Autodesk Inventor part; units mm, degrees
ref_plane "YZ Plane" through (0, 0, 0) normal (1, 0, 0) x (0, 1, 0)
ref_plane "XZ Plane" through (0, 0, 0) normal (0, 1, 0) x (-1, 0, 0)
ref_plane "XY Plane" through (0, 0, 0) normal (0, 0, 1) x (1, 0, 0)
sketch "Esboço1" plane through (0, 0, 0) normal (0, 1, 0) x (-1, 0, 0)
  circle A0 centre (0, 0) radius 15
  dimension "d0" = 30
extrude "Extrusão1" add sketch "Esboço1" along normal mid plane 21.5
fillet "Arredondamento1" radius 2 1 edges at (15, 10.75, 0)
sketch "Esboço2" plane through (0, -10.75, 0) normal (0, -1, 0) x (1, 0, 0)
  circle A0 centre (0, 0) radius 5
  dimension "d4" = 10
extrude "Extrusão2" cut sketch "Esboço2" against normal blind 10
sketch "Esboço3" plane through (0, 10.75, 0) normal (0, 1, 0) x (1, 0, 0)
  line L0 (2.5, -7.5) -> (-2.5, -7.5)
  line L1 (-2.5, -7.5) -> (-2.5, 7.5)
  line L2 (-2.5, 7.5) -> (2.5, 7.5)
  line L3 (2.5, 7.5) -> (2.5, -7.5)
  line L4 (2.5, -7.5) -> (-2.5, 7.5) construction
  line L5 (-2.5, -7.5) -> (2.5, 7.5) construction
  point P0 (0, 0)
  dimension "d7" = 5
  dimension "d8" = 15
extrude "Extrusão3" add sketch "Esboço3" along normal blind 44.25
fillet "Arredondamento2" radius 7.5 1 edges at (0, 55, 7.5)
fillet "Arredondamento3" radius 7.5 1 edges at (0, 55, -7.5)
fillet "Arredondamento4" radius 2 1 edges at (2.5, 10.75, 0)
fillet "Arredondamento5" radius 2 1 edges at (-2.5, 10.75, 0)
sketch "Esboço4" plane through (2.5, 47.5, 0) normal (1, 0, 0) x (0, 0, -1)
  line L0 (-7.5, -34.75) -> (-7.5, 0)
  line L1 (7.5, -34.75) -> (7.5, 0)
  line L2 (-7.5, 0) -> (7.5, 0) construction
  circle A0 centre (0, 0) radius 4
  point P0 (0, -47.5)
  dimension "d15" = 8
extrude "Extrusão4" add sketch "Esboço4" along normal blind 5.5
fillet "Arredondamento6" radius 0.5 1 edges at (8, 47.5, 4)
properties part number "Corpo do robo"
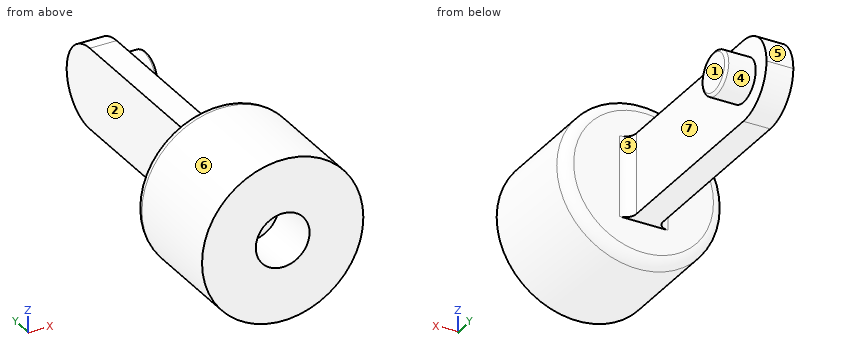
Could you check a few things on this model? Use its own coordinates, in mm. Face numbers are marked on the shaded views. A direction names the side the tool comes from. Coordinates: 2 decimals unless noted, no trailing zeros. Loops run counter-clockwise (first coordinate to the right, second up) from the corner with the lowest first, then second, coordinate; pieces in that order, holes last. Notation, with made-up numbers: (4, 70) -> (63, 70) arc R29 ccw to (63, 93) -> close; hole circle Ø11 at (-5, 31). An arc over 180 degrees is marked (long way). Answer in a Markdown table with one row per item.
(1) If I drill on probe 1 along Z at (x, y) = (0, -3); probe 2 along Y at (x, z) = (10.75, 3.5); probe 3 along Z at (x, y) = (-1, 18.5), over which ranges is the centre line in solid material (lowest first)?
Results found:
| item | result |
|---|---|
| probe 1 | z = -15 to -5, 5 to 15 |
| probe 2 | y = -10.75 to 10.75 |
| probe 3 | z = -7.5 to 7.5 |
(2) Will these pins go through, and if not, where does the flat tip stop? pin 1 Ø6 at (x, z) = (-2.5, 1.5) entering from +Y; pin 2 Ø5.5 at (y, z) = (46, 0.5) entering from +X; pin 3 Ø3 at (x, y) = (-12, 14) entering from -Z; pin 4 Ø3 at (x, z) = (-1.5, -2) entering from -Y.
Results found:
| item | result |
|---|---|
| pin 1 | stops at y = 55 |
| pin 2 | stops at x = 8 |
| pin 3 | passes through |
| pin 4 | stops at y = -0.75 |
(3) Imagine slicing it at B-B (y = 25.5). List the corners of the cut face in (x, z) for me, plus the area to 3 significant figures.
Results found:
| item | result |
|---|---|
| outline | (-2.5, -7.5) -> (2.5, -7.5) -> (2.5, 7.5) -> (-2.5, 7.5) -> close |
| area | 75.0 mm^2 |
(4) For the marked faces 1, 2, 3 and 4, which set-ups out of +Z, -Z, +X, -X, +Y, -Y let a thin tool reach every point of the face, with its end or its side?
Results found:
| item | result |
|---|---|
| face 1 | +Z, -Z, +X, +Y |
| face 2 | +Z, -Z, -X, +Y |
| face 3 | +Z, -Z, +X |
| face 4 | +X |
(5) Thinking about a two-plate mould opening in Y: for the marked faces 5, 6 and 7, which applies, released by +Y, released by -Y, zero draft, split by the parting line, or undercut?
Results found:
| item | result |
|---|---|
| face 5 | released by +Y |
| face 6 | zero draft |
| face 7 | undercut |
